```python
from build123d import *

# Parameters (mm, degrees)
BOSS_EXTRUDE1_DEPTH = 5


with BuildPart() as part:
    # Sketch1 → Boss-Extrude1 (new body)
    with BuildSketch(Plane(origin=(0, 0, -5), x_dir=(-1, 0, 0), z_dir=(0, 0, -1))):
        with BuildLine():
            Line((-25.000007614, -11.509619935), (-24.499994503, -60.010855227))
            ThreePointArc((-24.499994503, -60.010855227), (-15.782590077, -70.347575927), (-4.10890071, -63.523653936))
            Line((-4.10890071, -63.523653936), (16.891801465, -4.573510965))
            ThreePointArc((16.891801465, -4.573510965), (11.190796465, 13.454223259), (-7.573775299, 15.776184877))
            Line((-7.573775299, 15.776184877), (-28.686884347, 5.640277106))
            ThreePointArc((-28.686884347, 5.640277106), (-30.057470291, 5.16209183), (-31.500000671, 5.000002061))
            Line((-31.500000671, 5.000002061), (-308.500000671, 5.000002061))
            ThreePointArc((-308.500000671, 5.000002061), (-309.942531001, 5.162091818), (-311.313116903, 5.640277062))
            Line((-311.313116903, 5.640277062), (-332.426226108, 15.776184506))
            ThreePointArc((-332.426226108, 15.776184506), (-351.584092911, 13.117120589), (-356.591608654, -5.564936777))
            Line((-356.591608654, -5.564936777), (-325.67891256, -79.070456081))
            ThreePointArc((-325.67891256, -79.070456081), (-313.151079009, -85.106115073), (-305.620183213, -73.415888323))
            Line((-305.620183213, -73.415888323), (-314.961196041, -12.209189089))
            ThreePointArc((-314.961196041, -12.209189089), (-313.340441716, -7.161780706), (-308.500000492, -4.999997939))
            Line((-308.500000492, -4.999997939), (-31.500000492, -4.999997939))
            ThreePointArc((-31.500000492, -4.999997939), (-26.900405783, -6.907207011), (-25.000007614, -11.509619935))
        make_face()
        with BuildLine():
            Line((-31.500000492, -0.999997939), (-308.500000492, -0.999997939))
            ThreePointArc((-308.500000492, -0.999997939), (-316.350566349, -4.527292887), (-318.926606245, -12.739309227))
            Line((-318.926606245, -12.739309227), (-309.574399245, -74.019357929))
            ThreePointArc((-309.574399245, -74.019357929), (-314.236382275, -81.256164837), (-321.991707669, -77.519804575))
            Line((-321.991707669, -77.519804575), (-352.84288251, -4.160573117))
            ThreePointArc((-352.84288251, -4.160573117), (-348.883942975, 10.16492029), (-334.157374559, 12.170199891))
            Line((-334.157374559, 12.170199891), (-313.044265354, 2.034292448))
            ThreePointArc((-313.044265354, 2.034292448), (-310.830241974, 1.261839361), (-308.500000671, 1.000002061))
            Line((-308.500000671, 1.000002061), (-31.500000671, 1.000002061))
            ThreePointArc((-31.500000671, 1.000002061), (-29.169759288, 1.261839379), (-26.95573584, 2.034292518))
            Line((-26.95573584, 2.034292518), (-5.842626792, 12.170200289))
            ThreePointArc((-5.842626792, 12.170200289), (8.576792018, 10.425386169), (13.068119724, -3.387361226))
            Line((13.068119724, -3.387361226), (-7.876938579, -62.181308743))
            ThreePointArc((-7.876938579, -62.181308743), (-15.111557007, -66.404249616), (-20.499993004, -59.990382536))
            Line((-20.499993004, -59.990382536), (-21.000006097, -11.489149069))
            ThreePointArc((-21.000006097, -11.489149069), (-24.079215936, -4.071542072), (-31.500000492, -0.999997939))
        make_face(mode=Mode.SUBTRACT)
    extrude(amount=-BOSS_EXTRUDE1_DEPTH)


solid = part.part
```
Design review of the part built by this model. Coordinates are the model's own, in mm. A direction names the side the tool comes from. Round coordinates to 2 decimals unless told otherwise and drop trailing zeros. Order: outer loops, then holes, each group sorted by start corner. A loop starts at its lowest first (then second) coordinate and runs counter-clockwise, first axis right, second up. Notation, with made-up numbers: (21.5, 1) - (39.5, 1) arc R26 cw to (39.5, 32) - close; hole circle Ø8 at (37, 7.25). An arc over 180 degrees is marked (long way). One line per question, with ' | ' between items.
Item 1: Take a section at D-D, the plane x = 12.5. Write out the cut boundary in (y, z).
Checks:
outline: (-70.39, -5) - (-66.32, -5) - (-66.32, 0) - (-70.39, 0) - close; (8.97, -5) - (13.41, -5) - (13.41, 0) - (8.97, 0) - close
Item 2: For P1, Ø3, axis at x = 241.5, z = -0.5, coming from the -Y side; P2, Ø3, axis at y = -15.5, z = -3, coming from the -X side; P3, Ø1, axis at y = -24.5, z = -2.5, coming from the -X side, all flat-tipped, find the tip position at first contact; note any pin that passes through.
Checks:
P1: y = -5 | P2: x = -13.53 | P3: x = -9.97
Item 3: Take a section at B-B, the plane x = 155. Write out the cut boundary in (y, z).
Checks:
outline: (-5, -5) - (-1, -5) - (-1, 0) - (-5, 0) - close; (1, -5) - (5, -5) - (5, 0) - (1, 0) - close
Item 4: Machinability: for faces 1 (the face through (313.39, -7.22, -2.54)), 2 (the face through (185, -3, 0)), which of the approach directions +Z, -Z, +X, -X, +Y, -Y give a long, thin tool a straight path to every point of the face, cutting with its end or side? Answer none if there is none.
Checks:
face 1: +Z, -Z | face 2: +Z, +X, -X, +Y, -Y
Item 5: Take a section at C-C, the plane y = -34. Write out the cut boundary in (x, z).
Checks:
outline: (-6.41, -5) - (-2.16, -5) - (-2.16, 0) - (-6.41, 0) - close; (20.77, -5) - (24.77, -5) - (24.77, 0) - (20.77, 0) - close; (311.64, -5) - (315.68, -5) - (315.68, 0) - (311.64, 0) - close; (340.29, -5) - (344.63, -5) - (344.63, 0) - (340.29, 0) - close
Item 6: Wall thickness on line 1 (Y direction, x = 203.5, z = -0.85); line 2 (X direction, y = -64.5, z = -3.15); line 3 (X direction, y = -19.5, z = -4.45): over which ranges is each line inside the solid? List them lowest first. Write a range as [from, to].
Checks:
line 1: [-5, -1], [1, 5] | line 2: [4.51, 9.31], [18.69, 23.49], [306.98, 311.03], [327.47, 331.81] | line 3: [-11.57, -7.33], [20.92, 24.92], [313.85, 317.89], [346.39, 350.73]
